Here's how the part is built. I have some questions about the finished solid (model axes, mm). Round coordinates to 2 decimals unless told otherwise and drop trailing zeros. Write each loop counter-clockwise with the first axis right and the second up, starting at its lowest first coordinate (ties: lowest second). Pieces come first, ordered by that corner, then holes. Notation, with made-up numbers: M 32.5,6.5 L 44.5,6.5 A37 ccw 44.5,43.5 Z; hole C -36,-37.75 d8. An arc over 180 degrees is marked long. Write item = value, one per line. Start each with the question number.
(1) I want a section at B-B (x = 0.7). List the corners of the cut face in (y, z) for me, and give its area (3 significant figures).
(2) I want a section at C-C (y = 45). List the corners of the cut face in (x, z) for me, and give its area (3 significant figures).
(3) I want a section at A-A (z = 26.5). List the corners of the cut face in (x, y) for me, and give its area (3 significant figures).
(4) I want a section at D-D (y = 2). List the corners of the cut face in (x, z) for me.
(5) I need wall thicknesses on line 1 along Y through (x, z) = (0.75, 14); line 2 along Z through (x, y) = (0.85, 48.5); line 3 along Z through (x, y) = (0.7, 0). Which ranges of each line are inside material? Lowest first, please.
```python
from build123d import *

# Parameters (mm, degrees)
SKETCH_1_W          = 110.7
SKETCH_1_H          = 38.85
EXTRUDE_1_DEPTH     = 0.5
CUT_EXTRUDE_1_DEPTH = 110.343655509


with BuildPart() as part:
    # Эскиз1 → Бобышка-Вытянуть1 (new body)
    with BuildSketch(Plane(origin=(0.5, 0, 0), x_dir=(0, -1, 0), z_dir=(-1, 0, 0))):
        with Locations((-45.5, 22.825)):
            Rectangle(SKETCH_1_W, SKETCH_1_H)
    extrude(amount=-EXTRUDE_1_DEPTH)

    # Эскиз3 → Вырез-Вытянуть1 (cut, through all)
    with BuildSketch(Plane.ZY.offset(-0.5)):
        Polygon((30.006561442, 30.807083884), (-3.688047368, 30.807082411), (-3.688047368, 56.057082411), (30.006560338, 56.057083884), align=None)
        Polygon((30.106561442, -2.417922215), (-3.688047368, -2.417923692), (-3.688047368, 22.832076308), (30.106560338, 22.832077785), align=None)
    extrude(amount=-CUT_EXTRUDE_1_DEPTH, mode=Mode.SUBTRACT)


solid = part.part
```
Returned:
q1.outline = M -9.85,3.4 L -2.42,3.4 L -2.42,30.11 L 22.83,30.11 L 22.83,3.4 L 30.81,3.4 L 30.81,30.01 L 56.06,30.01 L 56.06,3.4 L 100.85,3.4 L 100.85,42.25 L -9.85,42.25 Z
q1.area = 2,950 mm²
q2.outline = M 0.5,30.01 L 1,30.01 L 1,42.25 L 0.5,42.25 Z
q2.area = 6.12 mm²
q3.outline = M 0.5,-9.85 L 1,-9.85 L 1,-2.42 L 0.5,-2.42 Z; M 0.5,22.83 L 1,22.83 L 1,30.81 L 0.5,30.81 Z; M 0.5,56.06 L 1,56.06 L 1,100.85 L 0.5,100.85 Z
q3.area = 30.1 mm²
q4.outline = M 0.5,30.11 L 1,30.11 L 1,42.25 L 0.5,42.25 Z
q5.line_1 = -9.85 to -2.42, 22.83 to 30.81, 56.06 to 100.85
q5.line_2 = 30.01 to 42.25
q5.line_3 = 30.11 to 42.25
